Part model, mm, in its own coordinate system. Coordinates: 2 decimals unless noted, no trailing zeros. Loops run counter-clockwise (first coordinate to the right, second up) from the corner with the lowest first, then second, coordinate; pieces in that order, holes last. Notation, with made-up numbers: (82, 14.25) - (131, 14.25) arc R15 ccw to (131, 29.25) - close; hole circle Ø1 at (-37, -23.5). An arc over 180 degrees is marked (long way). Use a Markdown table: item, result. Add a question column.
1) Probe probe 1 along Y at (x, z) = (0, 0.6); probe 2 along X at (y, z) = (3, 0.9); probe 3 along Y at (x, z) = (-23, 1.55). List the from-to ranges inside material, lowest first. Write a range as [from, to].
2) Drop a flat-ended pin along its axis: P1, Ø2.5, axis at x = -23, y = -25.98, coming from the +Z side. Give the stop position or say it passes through.
3) Band-saw the part on B-B (y = 25.98). Give the cut face in (x, z), plus the area to 3 significant figures.
4) Pull direction X, two halves, no side cores. Call faces 1 (the face through (-7.493, 0.33, 0.986)), 2 (the face through (8, 1, 0)), 3 (the face through (-30.55, -23.43, 0.99)): +X half, -X half, draft (parallel to the pull), parting line (faces both ways), or undercut.
5) Band-saw the part on A-A (x = 0). Give the cut face in (y, z).
6) Band-saw the part on C-C (x = -27.5). Give the cut face in (y, z), plus the area to 3 significant figures.
7) Band-saw the part on D-D (z = 1). Give the number of separate pieces and of enclosed holes in the cut face, plus the area to 3 significant figures.
from build123d import *

# Parameters (mm, degrees)
MODEL_R             = 38.5
MODEL_R_2           = 1.5
MODEL_R_3           = 5.5
MODEL_R_4           = 7.5
BOSS_EXTRUDE1_DEPTH = 2


with BuildPart() as part:
    # Model → Boss-Extrude1 (new body)
    with BuildSketch(Plane.XY):
        Circle(MODEL_R)
        with Locations((-23, 25.98)):
            Circle(MODEL_R_2, mode=Mode.SUBTRACT)
        with Locations((11.757144545, -32.646126143)):
            Circle(MODEL_R_2, mode=Mode.SUBTRACT)
        with Locations((11.757144545, 32.646126143)):
            Circle(MODEL_R_2, mode=Mode.SUBTRACT)
        with Locations((-23, -25.98)):
            Circle(MODEL_R_2, mode=Mode.SUBTRACT)
        with Locations((-25, 0)):
            Circle(MODEL_R_3, mode=Mode.SUBTRACT)
        with Locations((0, 25)):
            Circle(MODEL_R_3, mode=Mode.SUBTRACT)
        with Locations((0, -25)):
            Circle(MODEL_R_3, mode=Mode.SUBTRACT)
        with Locations((25, 0)):
            Circle(MODEL_R_3, mode=Mode.SUBTRACT)
        Circle(MODEL_R_4, mode=Mode.SUBTRACT)
    extrude(amount=BOSS_EXTRUDE1_DEPTH)


solid = part.part
Answer block:
| question | item | result |
|---|---|---|
| 1 | probe 1 | [-38.5, -30.5], [-19.5, -7.5], [7.5, 19.5], [30.5, 38.5] |
| 1 | probe 2 | [-38.38, -29.61], [-20.39, -6.87], [6.87, 20.39], [29.61, 38.38] |
| 1 | probe 3 | [-30.87, -27.48], [-24.48, -5.12], [5.12, 24.48], [27.48, 30.87] |
| 2 | P1 | through |
| 3 | outline | (-28.41, 0) - (-24.5, 0) - (-24.5, 2) - (-28.41, 2) - close; (-21.5, 0) - (-5.41, 0) - (-5.41, 2) - (-21.5, 2) - close; (5.41, 0) - (28.41, 0) - (28.41, 2) - (5.41, 2) - close |
| 3 | area | 86.0 mm2 |
| 4 | face 1 | undercut |
| 4 | face 2 | draft |
| 4 | face 3 | parting line |
| 5 | outline | (-38.5, 0) - (-30.5, 0) - (-30.5, 2) - (-38.5, 2) - close; (-19.5, 0) - (-7.5, 0) - (-7.5, 2) - (-19.5, 2) - close; (7.5, 0) - (19.5, 0) - (19.5, 2) - (7.5, 2) - close; (30.5, 0) - (38.5, 0) - (38.5, 2) - (30.5, 2) - close |
| 6 | outline | (-26.94, 0) - (-4.9, 0) - (-4.9, 2) - (-26.94, 2) - close; (4.9, 0) - (26.94, 0) - (26.94, 2) - (4.9, 2) - close |
| 6 | area | 88.2 mm2 |
| 7 | separate pieces | 1 |
| 7 | enclosed holes | 9 |
| 7 | area | 4,070 mm2 |
